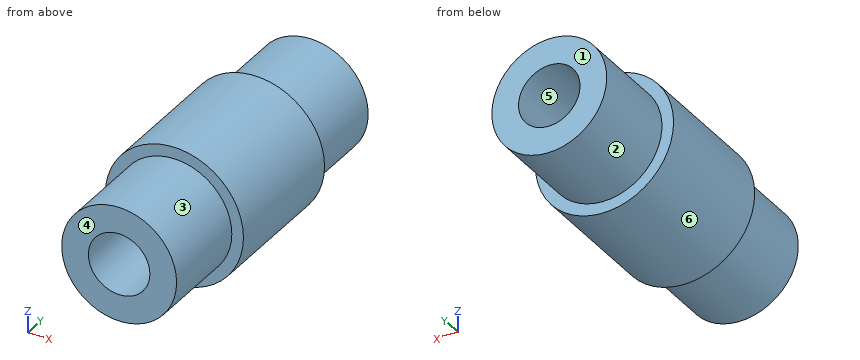
```python
from build123d import *

# Parameters (mm, degrees)
F0_R     = 5.95
F1_DEPTH = 5.8
F2_R     = 4.95
F3_DEPTH = 7.9
F5_R     = 2.65
F6_DEPTH = 35


with BuildPart() as f1:
    # F0 (on Front) → F1 (new body)
    with BuildSketch(Plane.XZ):
        Circle(F0_R)
    extrude(amount=F1_DEPTH)

    # F2 (on face) → F3 (join)
    with BuildSketch(Plane.XZ.offset(5.8)):
        Circle(F2_R)
    extrude(amount=F3_DEPTH)

    # F4: F1 across face


with BuildPart() as f1_1:
    add(f1.part)
    add(f1.part.mirror(Plane(origin=(0, 0, 0), x_dir=(1, 0, 0), z_dir=(0, 1, 0))))

    # F5 (on face) → F6 (cut)
    with BuildSketch(Plane.XZ.offset(13.7)):
        Circle(F5_R)
    extrude(amount=-F6_DEPTH, mode=Mode.SUBTRACT)


solid = f1_1.part
```
Verification items for the finished model (mm, model axes). Face numbers are marked on the shaded views. A direction names the side the tool comes from. Coordinates: 2 decimals unless noted, no trailing zeros. Order: outer loops, then holes, each group sorted by start corner. A loop starts at its lowest first (then second) coordinate and runs counter-clockwise, first axis right, second up. Notation, with made-up numbers: (-29, -11) -> (24, -11) arc R24 ccw to (24, -1) -> close; hole circle Ø5 at (55.25, -32). An arc over 180 degrees is marked (long way). Answer as CSV lines item,"result". Start each with the question number.
1) Cross-section at B-B, the plane x = 0. Record the boundary of the cut face in (y, z), then the cut area to 3 significant figures.
2) Cross-section at D-D, the plane z = 4.25. Record the boundary of the cut face in (x, y).
3) Cross-section at C-C, the plane y = -2. Record the boundary of the cut face in (x, z), then the cut area to 3 significant figures.
4) Material ranges on L1, parallel to Z at x = 0, y = 6.75; L2, parallel to Z at x = 0, y = -0.5; L3, parallel to Y at x = 3.75, z = -3.75, recorded low to high. Write a range as [from, to].
5) Gauge pin test, flat ends, axial feed: pin 1 Ø4 at (x, y) = (3, -10) entering from -Z; pin 2 Ø1.5 at (x, y) = (-0.5, -9.5) entering from -Z; pin 3 Ø4 at (y, z) = (-8.5, -1) entering from +X. Record the tip position at first contact, or that the pin passes through.
6) Cross-section at A-A, the plane z = 0. Record the boundary of the cut face in (x, y), then the cut area to 3 significant figures.
7) Set-up check for the marked faces 1, 2 and 3: record each of +Z, -Z, +X, -X, +Y, -Y from which the full face is reachable in a straight line by a thin tool's end or side.
8) Release check for a two-part mould opening along X. For the marked faces 4, 5 and 6 record: released by +X, released by -X, zero draft, split by the parting line, or undercut.
Conclusion:
1,outline,"(-13.7, -4.95) -> (-5.8, -4.95) -> (-5.8, -5.95) -> (5.8, -5.95) -> (5.8, -4.95) -> (13.7, -4.95) -> (13.7, -2.65) -> (-13.7, -2.65) -> close; (-13.7, 2.65) -> (13.7, 2.65) -> (13.7, 4.95) -> (5.8, 4.95) -> (5.8, 5.95) -> (-5.8, 5.95) -> (-5.8, 4.95) -> (-13.7, 4.95) -> close"
1,area,"149 mm²"
2,outline,"(-4.16, -5.8) -> (-2.54, -5.8) -> (-2.54, -13.7) -> (2.54, -13.7) -> (2.54, -5.8) -> (4.16, -5.8) -> (4.16, 5.8) -> (2.54, 5.8) -> (2.54, 13.7) -> (-2.54, 13.7) -> (-2.54, 5.8) -> (-4.16, 5.8) -> close"
3,outline,"circle Ø11.9 at (0, 0); hole circle Ø5.3 at (0, 0)"
3,area,"89.2 mm²"
4,L1,"z = [-4.95, -2.65], [2.65, 4.95]"
4,L2,"z = [-5.95, -2.65], [2.65, 5.95]"
4,L3,"y = [-5.8, 5.8]"
5,pin 1,"stops at z = -4.85"
5,pin 2,"stops at z = -4.95"
5,pin 3,"stops at x = 4.95"
6,outline,"(-5.95, -5.8) -> (-4.95, -5.8) -> (-4.95, -13.7) -> (-2.65, -13.7) -> (-2.65, 13.7) -> (-4.95, 13.7) -> (-4.95, 5.8) -> (-5.95, 5.8) -> close; (2.65, -13.7) -> (4.95, -13.7) -> (4.95, -5.8) -> (5.95, -5.8) -> (5.95, 5.8) -> (4.95, 5.8) -> (4.95, 13.7) -> (2.65, 13.7) -> close"
6,area,"149 mm²"
7,face 1,"+Z, -Z, +X, -X, +Y"
7,face 2,"+Y"
7,face 3,"-Y"
8,face 4,"zero draft"
8,face 5,"undercut"
8,face 6,"split by the parting line"
